Build history of the part. All positions in model axes, mm. Give positions to 0.01 mm unless a question says otherwise; leave off trailing zeros. Order: outer loops, then holes, each group sorted by start corner. A loop starts at its lowest first (then second) coordinate and runs counter-clockwise, first axis right, second up. Notation, with made-up numbers: (29.25, -22) -> (67.25, -22) arc R10 ccw to (67.25, -13) -> close; hole circle Ø5 at (88.25, 49). An arc over 180 degrees is marked (long way). One line per item, written item: value. Start each with the question number.
(1) Two-plate mould, pull along X, no slides. Class faces 1 (the cylindrical face through (94.508, 22.885, 0.386)), 2 (the flat face through (44, 30, 0)): +X half, -X half, draft (parallel to the pull), parting line (faces both ways), or undercut.
(2) Saw through at B-B on x = 63.5. Give the cut face in (y, z) (3 decimals), plus the area to 3 significant figures.
(3) Pin check, flat tips, straight feed: pin 1 (2 mm diameter, centred on x = 90.17, y = 5.334, fed in from -Z); pin 2 (4.5 mm diameter, centred on x = 63.5, y = 20.32, fed in from +Z). Stop position of each tip, or through.
(4) Probe line 1 (Y direction, x = 63.5, z = 0.4) (3 decimals); line 2 (Y direction, x = 90.17, z = 0.25); line 3 (X direction, y = 5, z = 0.5). List the from-to ranges inside material, lowest first.
(5) Saw through at D-D on y = 35. Give the cut face in (x, z) (3 decimals), plus the area to 3 significant figures.
(6) Saw through at A-A on y = 54.61. Give the cut face in (x, z) (3 decimals), plus the area to 3 significant figures.
(7) Saw through at C-C on z = 0.6. Give the cut face in (x, y) (3 decimals), plus the area to 3 significant figures.
```python
from build123d import *

# Parameters (mm, degrees)
F1_DEPTH = 0.762
F2_R     = 1.905
F3_DEPTH = 0.763
F4_R     = 1.35255
F5_DEPTH = 0.763


with BuildPart() as f1:
    # F0 (on Top) → F1 (new body)
    with BuildSketch(Plane.XY):
        Polygon((0, 76.2), (0, 0), (114.3, 0), (114.3, 27.432), (79.375, 27.432), (79.375, 49.022), (34.925, 49.022), (34.925, 76.2), align=None)
    extrude(amount=F1_DEPTH)

    # F2 (on face) → F3 (cut, through all)
    with BuildSketch(Plane.XY.offset(0.762)):
        with Locations((11.2014, 70.485)):
            Circle(F2_R)
        with Locations((2.8448, 54.61)):
            Circle(F2_R)
        with Locations((34.925, 8.9662)):
            Circle(F2_R)
        with Locations((63.5, 20.32)):
            Circle(F2_R)
    extrude(amount=-F3_DEPTH, mode=Mode.SUBTRACT)

    # F4 (on face) → F5 (cut, through all)
    with BuildSketch(Plane.XY.offset(0.762)):
        with Locations((93.218, 22.479)):
            Circle(F4_R)
        with Locations((90.17, 5.334)):
            Circle(F4_R)
    extrude(amount=-F5_DEPTH, mode=Mode.SUBTRACT)


solid = f1.part
```
Results below:
1. face 1: undercut
1. face 2: draft
2. outline: (0, 0) -> (18.415, 0) -> (18.415, 0.762) -> (0, 0.762) -> close; (22.225, 0) -> (49.022, 0) -> (49.022, 0.762) -> (22.225, 0.762) -> close
2. area: 34.5 mm²
3. pin 1: passes through
3. pin 2: stops at z = 0.76
4. line 1: y = 0 to 18.415, 22.225 to 49.022
4. line 2: y = 0 to 3.98, 6.69 to 27.43
4. line 3: x = 0 to 88.86, 91.48 to 114.3
5. outline: (0, 0) -> (79.375, 0) -> (79.375, 0.762) -> (0, 0.762) -> close
5. area: 60.5 mm²
6. outline: (0, 0) -> (0.94, 0) -> (0.94, 0.762) -> (0, 0.762) -> close; (4.75, 0) -> (34.925, 0) -> (34.925, 0.762) -> (4.75, 0.762) -> close
6. area: 23.7 mm²
7. outline: (0, 0) -> (114.3, 0) -> (114.3, 27.432) -> (79.375, 27.432) -> (79.375, 49.022) -> (34.925, 49.022) -> (34.925, 76.2) -> (0, 76.2) -> close; hole circle Ø3.81 at (2.845, 54.61); hole circle Ø3.81 at (11.201, 70.485); hole circle Ø3.81 at (34.925, 8.966); hole circle Ø3.81 at (63.5, 20.32); hole circle Ø2.705 at (90.17, 5.334); hole circle Ø2.705 at (93.218, 22.479)
7. area: 5,740 mm²
